from build123d import *

# Parameters (mm, degrees)
SKETCH1_W           = 127
SKETCH1_H           = 127
BOSS_EXTRUDE1_DEPTH = 38.1
SKETCH2_W           = 101.6
SKETCH2_H           = 9.525
CUT_EXTRUDE1_DEPTH  = 98.550550998
SKETCH3_R           = 3.175
CUT_EXTRUDE2_DEPTH  = 148.013128665


with BuildPart() as part:
    # Sketch1 → Boss-Extrude1 (new body)
    with BuildSketch(Plane(origin=(0, 0, 0), x_dir=(1, 0, 0), z_dir=(0, 1, 0))):
        Rectangle(SKETCH1_W, SKETCH1_H)
    extrude(amount=BOSS_EXTRUDE1_DEPTH)

    # Sketch2 → Cut-Extrude1 (cut, through all)
    with BuildSketch(Plane(origin=(0, 0, 0), x_dir=(-1, 0, 0), z_dir=(0, -1, 0))):
        Rectangle(SKETCH2_W, SKETCH2_H)
    extrude(amount=-CUT_EXTRUDE1_DEPTH, mode=Mode.SUBTRACT)

    # Sketch3 → Cut-Extrude2 (cut, through all)
    with BuildSketch(Plane.XY.offset(63.5)):
        with Locations((-25.4, 19.05)):
            Circle(SKETCH3_R)
        with Locations(Location((25.4, 19.05, 0), (0, 0, 180))):
            Circle(SKETCH3_R)
    extrude(amount=-CUT_EXTRUDE2_DEPTH, mode=Mode.SUBTRACT)


solid = part.part
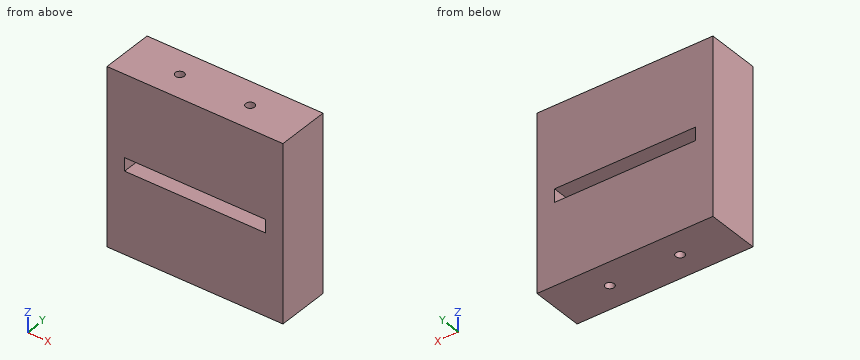
Build history of the part. All positions in model axes, mm. Coordinates: 2 decimals unless noted, no trailing zeros. Write each loop counter-clockwise with the first axis right and the second up, starting at its lowest first coordinate (ties: lowest second). Pieces come first, ordered by that corner, then holes.
(1) Cut at B-B on x = -14.5. List the corners of the cut face in (y, z), and give its area (3 significant figures).
(2) Cut at C-C on y = 19.05. List the corners of the cut face in (x, z) (1 decimal), and give its area (3 significant figures).
(3) Drill centre lines: line 1 (X direction, y = 19, z = 32); line 2 (Z direction, x = 5.5, y = 18.5); line 3 (X direction, y = 17.5, z = 58). Where is each one in solid material? Low to high.
(4) Pin check, flat tip, straight feed: pin 1 Ø10 at (x, y) = (-25.4, 19.05) entering from -Z. Stop position of the tip, or through.
(5) Cut at D-D on x = 25.4. List the corners of the cut face in (y, z) (1 decimal).
(6) Cut at A-A on y = 32. List the corners of the cut face in (x, z), and give its area (3 significant figures).
Working result:
1. outline: (0, -63.5) - (38.1, -63.5) - (38.1, -4.76) - (0, -4.76) - close; (0, 4.76) - (38.1, 4.76) - (38.1, 63.5) - (0, 63.5) - close
1. area: 4,480 mm2
2. outline: (-63.5, -63.5) - (-28.6, -63.5) - (-28.6, -4.8) - (-50.8, -4.8) - (-50.8, 4.8) - (-28.6, 4.8) - (-28.6, 63.5) - (-63.5, 63.5) - close; (-22.2, -63.5) - (22.2, -63.5) - (22.2, -4.8) - (-22.2, -4.8) - close; (-22.2, 4.8) - (22.2, 4.8) - (22.2, 63.5) - (-22.2, 63.5) - close; (28.6, -63.5) - (63.5, -63.5) - (63.5, 63.5) - (28.6, 63.5) - (28.6, 4.8) - (50.8, 4.8) - (50.8, -4.8) - (28.6, -4.8) - close
2. area: 13,700 mm2
3. line 1: x = -63.5 to -28.57, -22.23 to 22.23, 28.57 to 63.5
3. line 2: z = -63.5 to -4.76, 4.76 to 63.5
3. line 3: x = -63.5 to -28.17, -22.63 to 22.63, 28.17 to 63.5
4. pin 1: stops at z = -63.5
5. outline: (0, -63.5) - (15.9, -63.5) - (15.9, -4.8) - (0, -4.8) - close; (0, 4.8) - (15.9, 4.8) - (15.9, 63.5) - (0, 63.5) - close; (22.2, -63.5) - (38.1, -63.5) - (38.1, -4.8) - (22.2, -4.8) - close; (22.2, 4.8) - (38.1, 4.8) - (38.1, 63.5) - (22.2, 63.5) - close
6. outline: (-63.5, -63.5) - (63.5, -63.5) - (63.5, 63.5) - (-63.5, 63.5) - close; hole (-50.8, -4.76) - (50.8, -4.76) - (50.8, 4.76) - (-50.8, 4.76) - close
6. area: 15,200 mm2
